Model file for the job. Use its own axes, mm. Face numbers are marked on the shaded views. A direction names the side the tool comes from. Round coordinates to 2 decimals unless told otherwise and drop trailing zeros. Order: outer loops, then holes, each group sorted by start corner. A loop starts at its lowest first (then second) coordinate and runs counter-clockwise, first axis right, second up. Notation, with made-up numbers: (68, 0) - (112, 0) arc R24 ccw to (112, 15) - close; hole circle Ø9 at (-27.75, -20.5). An arc over 180 degrees is marked (long way). Use one line per item in the form item = value.
from build123d import *

# Parameters (mm, degrees)
F3_DEPTH = 6.35
F5_DEPTH = 25.4
F7_DEPTH = 3.175
F8_DEPTH = 3.302


with BuildPart() as f1:
    # F0 (on Front) → F1 (revolve)
    with BuildSketch(Plane.XZ):
        Polygon((59.4741, 0), (0, 0), (0, -12.7508), (50.8, -12.7508), (50.8, -5.626218), (59.4741, -3.302), align=None)
    revolve(axis=Axis((0, 0, -6.3754), (0, 0, -1)))

    # F2 (on face) → F3 (cut)
    with BuildSketch(Plane.XY):
        with BuildLine():
            Line((-40.64, -4.826), (-38.1, -4.826))
            ThreePointArc((-38.1, -4.826), (-33.274, 0), (-38.1, 4.826))
            Line((-38.1, 4.826), (-40.64, 4.826))
            ThreePointArc((-40.64, 4.826), (-45.466, 0), (-40.64, -4.826))
        make_face()
    extrude(amount=-F3_DEPTH, mode=Mode.SUBTRACT)

    # F4 (on face) → F5 (cut)
    with BuildSketch(Plane.XY):
        with BuildLine():
            ThreePointArc((-59.346964, -0.127), (-59.3471, 0), (-59.346964, 0.127))
            Line((-59.346964, 0.127), (-59.4741, 0.127))
            Line((-59.4741, 0.127), (-59.4741, -0.127))
            Line((-59.4741, -0.127), (-59.346964, -0.127))
        make_face()
    extrude(amount=-F5_DEPTH, mode=Mode.SUBTRACT)

    # F6 (on face) → F7 (cut)
    with BuildSketch(Plane(origin=(0, 0, -12.7508), x_dir=(1, 0, 0), z_dir=(0, 0, -1))):
        with BuildLine():
            Line((3.169708, -25.174637), (3.169708, -0.00022))
            Line((3.169708, -0.00022), (3.169708, 25.174198))
            ThreePointArc((3.169708, 25.174198), (0, 28.532442), (-3.169708, 25.174198))
            Line((-3.169708, 25.174198), (-3.169708, -0.00022))
            Line((-3.169708, -0.00022), (-3.169708, -25.174637))
            ThreePointArc((-3.169708, -25.174637), (0, -28.532881), (3.169708, -25.174637))
        make_face()
    extrude(amount=-F7_DEPTH, mode=Mode.SUBTRACT)

    # F6 (on face) → F8 (cut)
    with BuildSketch(Plane(origin=(0, 0, -12.7508), x_dir=(1, 0, 0), z_dir=(0, 0, -1))):
        with BuildLine():
            Line((3.169708, -25.174637), (3.169708, -0.00022))
            Line((3.169708, -0.00022), (3.169708, 25.174198))
            ThreePointArc((3.169708, 25.174198), (0, 28.532442), (-3.169708, 25.174198))
            Line((-3.169708, 25.174198), (-3.169708, -0.00022))
            Line((-3.169708, -0.00022), (-3.169708, -25.174637))
            ThreePointArc((-3.169708, -25.174637), (0, -28.532881), (3.169708, -25.174637))
        make_face()
    extrude(amount=-F8_DEPTH, mode=Mode.SUBTRACT)


solid = f1.part
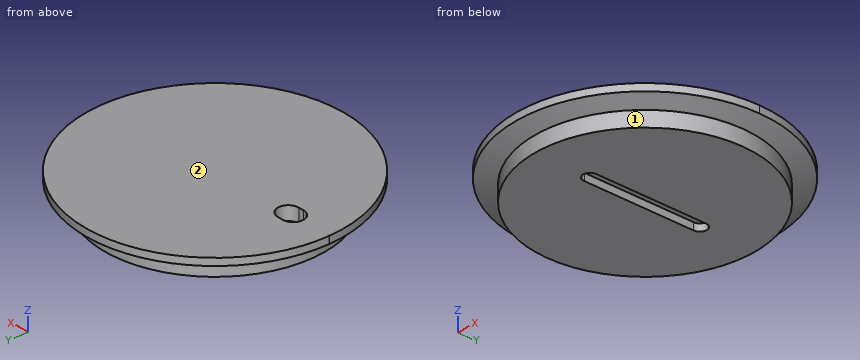
(1) Tool access for the marked faces 1 and 2: list every direction of +Z, -Z, +X, -X, +Y, -Y with a clear straight run to the whole face (end or side of a thin tool).
Report:
face_1 = -Z
face_2 = +Z, +X, -X, +Y, -Y
(2) Pin check, flat tips, straight feed: pin 1 (1.7 mm diameter, centred on y = -2.5, z = -10.5, fed in from +X); pin 2 (2 mm diameter, centred on x = -39, z = -2.5, fed in from -Y); pin 3 (4 mm diameter, centred on x = -30.5, z = -8.5, fed in from +Y). Stop position of each tip, or through.
Report:
pin_1 = 50.77
pin_2 = -45.75
pin_3 = 42.05
(3) Slice it at A-A on x = 0. Give the cut face in (y, z).
Report:
outline = (-59.47, -3.3) - (-50.8, -5.63) - (-50.8, -12.75) - (-28.53, -12.75) - (-28.53, -9.45) - (28.53, -9.45) - (28.53, -12.75) - (50.8, -12.75) - (50.8, -5.63) - (59.47, -3.3) - (59.47, 0) - (-59.47, 0) - close
(4) Probe probe 1 along Z at (x, y) = (2, 21); probe 2 along X at (y, z) = (7.5, -11); probe 3 along X at (y, z) = (-9, -10). List the from-to ranges inside material, lowest first. Write a range as [from, to].
Report:
probe_1 = [-9.45, 0]
probe_2 = [-50.24, -3.17], [3.17, 50.24]
probe_3 = [-50, -3.17], [3.17, 50]
